Read the model definition and answer for the solid it produces. Units are mm, in the model's axes. Face numbers are marked on the shaded views. A direction names the side the tool comes from. Give positions to 0.01 mm unless a question says otherwise; leave off trailing zeros. Write each loop counter-clockwise with the first axis right and the second up, starting at its lowest first coordinate (ties: lowest second). Pieces come first, ordered by that corner, then holes. Notation, with made-up numbers: (-6.5, 83.25) -> (49.5, 83.25) arc R24 ccw to (49.5, 120.25) -> close; hole circle Ø5 at (32.25, 30.5). An arc over 180 degrees is marked (long way). Use a Markdown table: item, result.
from build123d import *

# Parameters (mm, degrees)
SKETCH_2_R      = 4
EXTRUDE_1_DEPTH = 8.2
SKETCH_4_R      = 0.5
EXTRUDE_2_DEPTH = 7
SKETCH_5_R      = 1.5
EXTRUDE_3_DEPTH = 1
SKETCH_6_W      = 1.5
SKETCH_6_H      = 4
EXTRUDE_4_DEPTH = 5
EXTRUDE_5_DEPTH = 1
FILLET_1_R      = 10
SKETCH_8_R      = 2
EXTRUDE_6_DEPTH = 0.5


with BuildPart() as part:
    # 草图2 → 凸台-拉伸1 (new body)
    with BuildSketch(Plane.XY):
        Circle(SKETCH_2_R)
    extrude(amount=EXTRUDE_1_DEPTH)

    # 草图4 → 凸台-拉伸2 (add)
    with BuildSketch(Plane.XY.offset(8.2)):
        Circle(SKETCH_4_R)
    extrude(amount=EXTRUDE_2_DEPTH)

    # 草图5 → 凸台-拉伸3 (add)
    with BuildSketch(Plane.XY.offset(8.2)):
        Circle(SKETCH_5_R)
    extrude(amount=EXTRUDE_3_DEPTH)

    # 草图6 → 凸台-拉伸4 (add)
    with BuildSketch(Plane(origin=(0, 0, 0), x_dir=(0, 0, -1), z_dir=(1, 0, 0))):
        with Locations((-3.75, 0)):
            Rectangle(SKETCH_6_W, SKETCH_6_H)
    extrude(amount=EXTRUDE_4_DEPTH)

    # 草图7 → 凸台-拉伸5 (add)
    with BuildSketch(Plane.XY.offset(8.2)):
        with BuildLine():
            Line((4, 0), (1.5, 0))
            ThreePointArc((1.5, 0), (0, -1.5), (-1.5, 0))
            Line((-1.5, 0), (-4, 0))
            ThreePointArc((-4, 0), (-3.60468391, -1.733855216), (-2.496873044, -3.125))
            ThreePointArc((-2.496873044, -3.125), (-1.69373638, -3.623707642), (-0.79598995, -3.92))
            ThreePointArc((-0.79598995, -3.92), (0, -3.2), (0.79598995, -3.92))
            ThreePointArc((0.79598995, -3.92), (1.69373638, -3.623707642), (2.496873044, -3.125))
            ThreePointArc((2.496873044, -3.125), (3.60468391, -1.733855216), (4, 0))
        make_face()
        with BuildLine():
            ThreePointArc((-2.496873044, -3.125), (0, -5.5), (2.496873044, -3.125))
            ThreePointArc((2.496873044, -3.125), (1.69373638, -3.623707642), (0.79598995, -3.92))
            ThreePointArc((0.79598995, -3.92), (0.798996858, -3.95994978), (0.8, -4))
            ThreePointArc((0.8, -4), (-0.04005022, -4.798996858), (-0.79598995, -3.92))
            ThreePointArc((-0.79598995, -3.92), (-1.69373638, -3.623707642), (-2.496873044, -3.125))
        make_face()
        with BuildLine():
            ThreePointArc((-1.5, 0), (0, 1.5), (1.5, 0))
            Line((1.5, 0), (4, 0))
            ThreePointArc((4, 0), (3.60468391, 1.733855216), (2.496873044, 3.125))
            ThreePointArc((2.496873044, 3.125), (1.69373638, 3.623707642), (0.79598995, 3.92))
            ThreePointArc((0.79598995, 3.92), (0, 3.2), (-0.79598995, 3.92))
            ThreePointArc((-0.79598995, 3.92), (-1.69373638, 3.623707642), (-2.496873044, 3.125))
            ThreePointArc((-2.496873044, 3.125), (-3.60468391, 1.733855216), (-4, 0))
            Line((-4, 0), (-1.5, 0))
        make_face()
        with BuildLine():
            ThreePointArc((0.79598995, 3.92), (1.69373638, 3.623707642), (2.496873044, 3.125))
            ThreePointArc((2.496873044, 3.125), (0, 5.5), (-2.496873044, 3.125))
            ThreePointArc((-2.496873044, 3.125), (-1.69373638, 3.623707642), (-0.79598995, 3.92))
            ThreePointArc((-0.79598995, 3.92), (-0.04005022, 4.798996858), (0.8, 4))
            ThreePointArc((0.8, 4), (0.798996858, 3.95994978), (0.79598995, 3.92))
        make_face()
    extrude(amount=EXTRUDE_5_DEPTH)

    # 圆角1
    # the kernel refuses this fillet: 10 mm, written as the material it adds along each edge
    with BuildSketch(Plane(origin=(2.496873044, 3.125, 8.2), x_dir=(0.6874097542343248, -0.7262698050886497, 0), z_dir=(0, 0, 1)), Plane(origin=(-2.496873044, -3.125, 8.2), x_dir=(-0.6874097542343238, 0.7262698050886505, 0), z_dir=(0, 0, 1))) as fillet_1_piece_1:
        with BuildLine():
            CenterArc((2.489482148, 9.903897453), FILLET_1_R, 250.779418195, 11.270831285)
            ThreePointArc((-0.802576499, 0.461315716), (-0.379749812, 0.26812947), (0, 0))
            ThreePointArc((0, 0), (0.553218255, 0.038441019), (1.10643651, 0))
        make_face()
    extrude(amount=1)
    with BuildSketch(Plane(origin=(-2.496873044, 3.125, 8.2), x_dir=(-0.6874097542343243, -0.7262698050886502, 0), z_dir=(0, 0, 1)), Plane(origin=(2.496873044, -3.125, 8.2), x_dir=(0.6874097542343256, 0.7262698050886488, 0), z_dir=(0, 0, 1))) as fillet_1_piece_2:
        with BuildLine():
            CenterArc((2.489482148, -9.903897453), FILLET_1_R, 97.94975052, 11.270831285)
            ThreePointArc((-0.802576499, -0.461315716), (-0.379749812, -0.26812947), (0, 0))
            ThreePointArc((0, 0), (0.553218255, -0.038441019), (1.10643651, 0))
        make_face()
    extrude(amount=1)

    # 草图8 → 凸台-拉伸6 (add)
    with BuildSketch(Plane.XY.offset(9.2)):
        Circle(SKETCH_8_R)
    extrude(amount=EXTRUDE_6_DEPTH)


solid = part.part
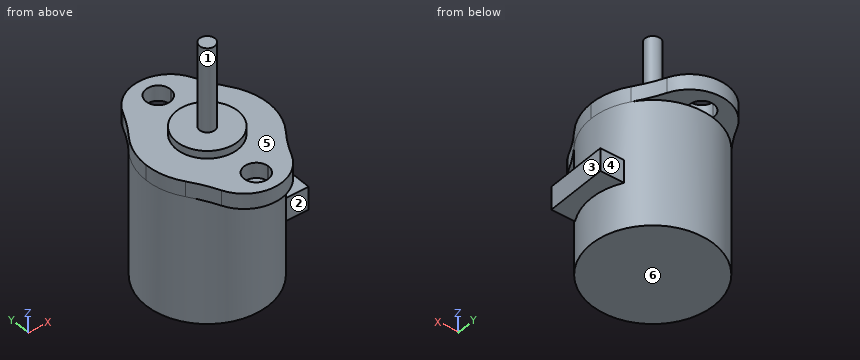
Item 1: Each of these flat-tipped pins is pushed along its axis until it touches: P1, Ø0.6, axis at x = 0.5, y = 3.5, coming from the +Z side; P2, Ø0.8, axis at x = 4.5, z = 3.5, coming from the -Y side; P3, Ø5, axis at y = -4.5, z = 6.5, coming from the +X side. Where does it stop, or does it pass through?
Return value:
| item | result |
|---|---|
| P1 | z = 9.2 |
| P2 | y = -2 |
| P3 | x = 3.46 |
Item 2: A cutting plane is placed at A-A (x = 0). Give the vertices of the cut face in (y, z), then the cut area to 3 significant figures.
Return value:
| item | result |
|---|---|
| outline | (-5.5, 8.2) -> (-4.8, 8.2) -> (-4.8, 9.2) -> (-5.5, 9.2) -> close; (-4, 0) -> (4, 0) -> (4, 8.2) -> (3.2, 8.2) -> (3.2, 9.2) -> (2, 9.2) -> (2, 9.7) -> (0.5, 9.7) -> (0.5, 15.2) -> (-0.5, 15.2) -> (-0.5, 9.7) -> (-2, 9.7) -> (-2, 9.2) -> (-3.2, 9.2) -> (-3.2, 8.2) -> (-4, 8.2) -> close; (4.8, 8.2) -> (5.5, 8.2) -> (5.5, 9.2) -> (4.8, 9.2) -> close |
| area | 80.9 mm^2 |
Item 3: A cutting plane is placed at B-B (y = -3.5). Give the vertices of the cut face in (x, z).
Return value:
| item | result |
|---|---|
| outline | (-2.53, 8.2) -> (-1.94, 8.2) -> (-1.94, 0) -> (1.94, 0) -> (1.94, 8.2) -> (2.53, 8.2) -> (2.53, 9.2) -> (0.62, 9.2) -> (0.62, 8.2) -> (-0.62, 8.2) -> (-0.62, 9.2) -> (-2.53, 9.2) -> close |
Item 4: Straight lines are drawn through the part: line 1 along Z through (x, y) = (-1.75, -4.25); line 2 along Z through (x, y) = (-2, 3); line 3 along X through (y, z) = (-2.75, 8.5). For each, find the intervals that lie inside material, in ascending order. Write a range as [from, to].
Return value:
| item | result |
|---|---|
| line 1 | [8.2, 9.2] |
| line 2 | [0, 9.2] |
| line 3 | [-2.97, 2.97] |
Item 5: A cutting plane is placed at D-D (x = 3). Give the vertices of the cut face in (y, z).
Return value:
| item | result |
|---|---|
| outline | (-2.7, 8.2) -> (-2.65, 8.2) -> (-2.65, 0) -> (2.65, 0) -> (2.65, 8.2) -> (2.7, 8.2) -> (2.7, 9.2) -> (-2.7, 9.2) -> close |
Item 6: A tool of negligible diameter and unlimited length cuts with its end or side. For the marked faces 4, 5 and 6, from which of +Z, -Z, +X, -X, +Y, -Y can it reach the whole face along a straight path? Write none if from no direction.
Return value:
| item | result |
|---|---|
| face 4 | +Z, -Z, +X, +Y |
| face 5 | +Z |
| face 6 | -Z, +X, -X, +Y, -Y |
Item 7: A cutting plane is placed at C-C (z = 12.25). Give the vertices of the cut face in (x, y), then the cut area to 3 significant figures.
Return value:
| item | result |
|---|---|
| outline | circle Ø1 at (0, 0) |
| area | 0.785 mm^2 |
Item 8: For a pull along X with two mould halves and no side action, classify the marked faces 1, 2 and 3 as +X half, -X half, draft (parallel to the pull), parting line (faces both ways), or undercut.
Return value:
| item | result |
|---|---|
| face 1 | parting line |
| face 2 | draft |
| face 3 | +X half |
